```python
from build123d import *

# Parameters (mm, degrees)
BOSS_EXTRUDE1_DEPTH = 7.9375
SKETCH3_R           = 2.7559
CUT_EXTRUDE1_DEPTH  = 3.81
CUT_EXTRUDE2_REACH  = 11.398
SKETCH4_R           = 1.7526
SKETCH5_R           = 6.35
BOSS_EXTRUDE2_DEPTH = 1.5875


with BuildPart() as part:
    # Sketch1 → Boss-Extrude1 (new body)
    with BuildSketch(Plane(origin=(0, 0, 0), x_dir=(1, 0, 0), z_dir=(0, 1, 0))):
        with BuildLine():
            ThreePointArc((-6.35, 0), (0, -6.35), (6.35, 0))
            Line((6.35, 0), (6.35, 6.858))
            Line((6.35, 6.858), (-6.35, 6.858))
            Line((-6.35, 6.858), (-6.35, 0))
        make_face()
        with BuildLine():
            Line((-2.032, 2.439590334), (2.032, 2.439590334))
            ThreePointArc((2.032, 2.439590334), (0, -3.175), (-2.032, 2.439590334))
        make_face(mode=Mode.SUBTRACT)
    extrude(amount=BOSS_EXTRUDE1_DEPTH)

    # Sketch3 → Cut-Extrude1 (cut)
    with BuildSketch(Plane(origin=(0, 0, -6.858), x_dir=(-1, 0, 0), z_dir=(0, 0, -1))):
        with Locations((0, 3.96875)):
            Circle(SKETCH3_R)
    extrude(amount=-CUT_EXTRUDE1_DEPTH, mode=Mode.SUBTRACT)

    # Sketch4 → Cut-Extrude2 (cut, up to next)
    with BuildSketch(Plane(origin=(0, 0, -3.048), x_dir=(-1, 0, 0), z_dir=(0, 0, -1)), mode=Mode.PRIVATE) as cut_extrude2_sk1:
        with Locations((0, 3.96875)):
            Circle(SKETCH4_R)
    cut_extrude2_tool1 = extrude(cut_extrude2_sk1.sketch, amount=-CUT_EXTRUDE2_REACH, mode=Mode.PRIVATE) & part.part
    add(cut_extrude2_tool1.solids().sort_by_distance((0, 3.96875, -3.048))[0], mode=Mode.SUBTRACT)

    # Sketch5 → Boss-Extrude2 (add)
    with BuildSketch(Plane(origin=(0, 7.9375, 0), x_dir=(1, 0, 0), z_dir=(0, 1, 0))):
        Circle(SKETCH5_R)
        with BuildLine():
            Line((-2.032, 2.439590334), (2.032, 2.439590334))
            ThreePointArc((2.032, 2.439590334), (0, -3.175), (-2.032, 2.439590334))
        make_face(mode=Mode.SUBTRACT)
    extrude(amount=BOSS_EXTRUDE2_DEPTH)


solid = part.part
```
Input: part model. Units: mm. Frame: model coordinates. A direction names the side the tool comes from. Give positions to 0.01 mm unless a question says otherwise; leave off trailing zeros. Write each loop counter-clockwise with the first axis right and the second up, starting at its lowest first coordinate (ties: lowest second). Pieces come first, ordered by that corner, then holes. Notation, with made-up numbers: (54, 13) - (62, 13) arc R25 cw to (62, 40) - close; hole circle Ø7 at (-27.75, 46). An arc over 180 degrees is marked (long way). Write item = value, one per line. Start each with the question number.
1. Access query for faces 4 (the cylindrical face through (2.93, 4.696, 5.634)), 5 (the flat face through (0, 9.525, -3)), 6 (the flat face through (0, 6, -2.44)), 7 (the cylindrical face through (0.6, 1.28, -4.98)). Directions: +Z, -Z, +X, -X, +Y, -Y. A direction counts if a zero-diameter tool reaches every point of the face in a straight line with its end or side. Return the directions, or none.
2. First-contact query: pin 1 Ø3 at (x, y) = (2, 3) entering from +Z; pin 2 Ø5 at (x, y) = (0, 3.97) entering from -Z; pin 3 Ø3 at (x, y) = (0, 3.97) entering from -Z. Flat tips, straight axial feed; report the tip coordinate or a pass-through.
3. Ray query, L1, parallel to Y at x = 0, z = -6 (3 decimals); L2, parallel to X at y = 8.75, z = -5.5; L3, parallel to X at y = 4.5, z = -2. Return the intervals inside material, ascending.
4. Section query A-A, the plane x = 0. Count the separate pieces of the cut face and the enclosed holes in it, then the cut area to 3 significant figures.
5. Mould query, pull axis X, two halves, no side actions, for faces 1 (the flat face through (-6.35, 4, -3)), 2 (the flat face through (0, 7.938, -6.7)), 3 (the flat face through (-2, 4, -3.048)). Classes: released by +X, released by -X, zero draft, split by the parting line, or undercut.
6. Section query D-D, the plane x = 2.5. Output: boundary loops of the cut face in (y, z) (1 decimal).
Check sheet entries:
q1.face_4 = +Y
q1.face_5 = +Z, -Z, +X, -X, +Y
q1.face_6 = +Y, -Y
q1.face_7 = -Z
q2.pin_1 = 6.33
q2.pin_2 = -3.05
q2.pin_3 = 2.8
q3.L1 = 0 to 1.213, 6.725 to 9.525
q3.L2 = -3.17 to 3.17
q3.L3 = -6.35 to -2.47, 2.47 to 6.35
q4.separate_pieces = 3
q4.enclosed_holes = 0
q4.area = 48.4 mm2
q5.face_1 = released by -X
q5.face_2 = zero draft
q5.face_3 = undercut
q6.outline = (0, -6.9) - (2.8, -6.9) - (2.8, -3) - (5.1, -3) - (5.1, -6.9) - (7.9, -6.9) - (7.9, -5.8) - (9.5, -5.8) - (9.5, -2) - (0, -2) - close; (0, 2) - (9.5, 2) - (9.5, 5.8) - (0, 5.8) - close
